from build123d import *

# Parameters (mm, degrees)
ESBO_O1_R                   = 16
RESSALTO_EXTRUS_O1_DEPTH    = 42
CASCA1_T                    = -5
ESBO_O3_R                   = 2
ESBO_O3_W                   = 60
ESBO_O3_H                   = 15
CORTE_EXTRUS_O1_DEPTH       = 5
ESBO_O4_R                   = 29
ESBO_O4_R_2                 = 24
RESSALTO_EXTRUS_O2_DEPTH    = 9
ESBO_O5_R                   = 9
CORTE_EXTRUS_O2_DEPTH       = 5
ESBO_O6_R                   = 14.5
ESBO_O6_R_2                 = 11.5
RESSALTO_EXTRUS_O3_DEPTH    = 6
NERVURA1_REACH              = 150.27
ESBO_O7_WALLS_W             = 304.540047886
ESBO_O7_WALLS_H             = 10
ESBO_O7_WALLS_W_2           = 10
ESBO_O7_WALLS_H_2           = 304.540047886
NERVURA2_REACH              = 150.866
ESBO_O8_WALLS_W             = 320.231422594
ESBO_O8_WALLS_H             = 10
ESBO_O8_WALLS_W_2           = 10
ESBO_O8_WALLS_H_2           = 400.231422594
ESBO_O8_WALLS_H_3           = 336.231422594
CORTE_EXTRUS_O3_DEPTH       = 5
ESBO_O10_R                  = 1.2
CORTE_EXTRUS_O4_DEPTH       = 5
RESSALTO_EXTRUS_O4_DEPTH    = 4
FILETE1_R                   = 1.5
PADR_O_LINEAR1_COUNT        = 3
PADR_O_LINEAR1_PITCH        = 65
FILETE1_OF_PADR_O_LINEAR1_R = 1.5


with BuildPart() as part:
    # Esboço1 → Ressalto-extrusão1 (new body)
    with BuildSketch(Plane.XY):
        with BuildLine():
            Line((-40, -100), (-40, 100))
            Line((-40, 100), (40, 100))
            Line((40, 100), (40, -100))
            ThreePointArc((40, -100), (0, -140), (-40, -100))
        make_face()
        with Locations(Location((0, -100, 0), (0, 0, 180))):
            Circle(ESBO_O1_R, mode=Mode.SUBTRACT)
    extrude(amount=RESSALTO_EXTRUS_O1_DEPTH)

    # Casca1
    casca1_openings = [part.faces().sort_by_distance(p)[0] for p in [
        (0, -12.059912395, 42),
        (16, -100, 21),
    ]]
    offset(amount=CASCA1_T, openings=casca1_openings, kind=Kind.INTERSECTION)

    # Esboço3 → Corte-extrusão1 (cut)
    with BuildSketch(Plane(origin=(0, 100, 0), x_dir=(1, 0, 0), z_dir=(0, 1, 0))):
        with Locations(Location((25, -33.5, 0), (0, 0, 270))):
            Circle(ESBO_O3_R)
        with Locations(Location((-25, -33.5, 0), (0, 0, 270))):
            Circle(ESBO_O3_R)
        with Locations(Location((-25, -8.5, 0), (0, 0, 270))):
            Circle(ESBO_O3_R)
        with Locations(Location((25, -8.5, 0), (0, 0, 270))):
            Circle(ESBO_O3_R)
        with Locations((0, -21)):
            Rectangle(ESBO_O3_W, ESBO_O3_H)
    extrude(amount=-CORTE_EXTRUS_O1_DEPTH, mode=Mode.SUBTRACT)

    # Esboço4 → Ressalto-extrusão2 (add)
    with BuildSketch(Plane.XY.offset(5)):
        with Locations((0, -100)):
            Circle(ESBO_O4_R)
        with Locations((0, -100)):
            Circle(ESBO_O4_R_2, mode=Mode.SUBTRACT)
    extrude(amount=RESSALTO_EXTRUS_O2_DEPTH)

    # Esboço5 → Corte-extrusão2 (cut)
    with BuildSketch(Plane.XY.offset(5)):
        with Locations((0, -20)):
            Circle(ESBO_O5_R)
    extrude(amount=-CORTE_EXTRUS_O2_DEPTH, mode=Mode.SUBTRACT)

    # Esboço6 → Ressalto-extrusão3 (add)
    with BuildSketch(Plane.XY.offset(5)):
        with Locations((0, -20)):
            Circle(ESBO_O6_R)
        with Locations((0, -20)):
            Circle(ESBO_O6_R_2, mode=Mode.SUBTRACT)
    extrude(amount=RESSALTO_EXTRUS_O3_DEPTH)

    # Esboço7 walls → Nervura1 (add, up to next)
    with BuildSketch(Plane.XY.offset(14), mode=Mode.PRIVATE) as nervura1_sk1:
        with Locations((32, -100)):
            Rectangle(ESBO_O7_WALLS_W, ESBO_O7_WALLS_H)
    nervura1_tool1 = extrude(nervura1_sk1.sketch, amount=-NERVURA1_REACH, mode=Mode.PRIVATE) - part.part
    # Esboço7 walls → Nervura1 (add, up to next)
    with BuildSketch(Plane.XY.offset(14), mode=Mode.PRIVATE) as nervura1_sk2:
        with Locations((-32, -100)):
            Rectangle(ESBO_O7_WALLS_W, ESBO_O7_WALLS_H)
    nervura1_tool2 = extrude(nervura1_sk2.sketch, amount=-NERVURA1_REACH, mode=Mode.PRIVATE) - part.part
    # Esboço7 walls → Nervura1 (add, up to next)
    with BuildSketch(Plane.XY.offset(14), mode=Mode.PRIVATE) as nervura1_sk3:
        with Locations((0, -132)):
            Rectangle(ESBO_O7_WALLS_W_2, ESBO_O7_WALLS_H_2)
    nervura1_tool3 = extrude(nervura1_sk3.sketch, amount=-NERVURA1_REACH, mode=Mode.PRIVATE) - part.part
    add(nervura1_tool1.solids().sort_by_distance((32, -100, 14))[0])
    add(nervura1_tool2.solids().sort_by_distance((-32, -100, 14))[0])
    add(nervura1_tool3.solids().sort_by_distance((0, -132, 14))[0])

    # Esboço8 walls → Nervura2 (add, up to next)
    with BuildSketch(Plane.XY.offset(11), mode=Mode.PRIVATE) as nervura2_sk1:
        with Locations((24.75, -20)):
            Rectangle(ESBO_O8_WALLS_W, ESBO_O8_WALLS_H)
    nervura2_tool1 = extrude(nervura2_sk1.sketch, amount=-NERVURA2_REACH, mode=Mode.PRIVATE) - part.part
    # Esboço8 walls → Nervura2 (add, up to next)
    with BuildSketch(Plane.XY.offset(11), mode=Mode.PRIVATE) as nervura2_sk2:
        with Locations((-24.75, -20)):
            Rectangle(ESBO_O8_WALLS_W, ESBO_O8_WALLS_H)
    nervura2_tool2 = extrude(nervura2_sk2.sketch, amount=-NERVURA2_REACH, mode=Mode.PRIVATE) - part.part
    # Esboço8 walls → Nervura2 (add, up to next)
    with BuildSketch(Plane.XY.offset(11), mode=Mode.PRIVATE) as nervura2_sk3:
        with Locations((0, 44.75)):
            Rectangle(ESBO_O8_WALLS_W_2, ESBO_O8_WALLS_H_2)
    nervura2_tool3 = extrude(nervura2_sk3.sketch, amount=-NERVURA2_REACH, mode=Mode.PRIVATE) - part.part
    # Esboço8 walls → Nervura2 (add, up to next)
    with BuildSketch(Plane.XY.offset(11), mode=Mode.PRIVATE) as nervura2_sk4:
        with Locations((0, -52.75)):
            Rectangle(ESBO_O8_WALLS_W_2, ESBO_O8_WALLS_H_3)
    nervura2_tool4 = extrude(nervura2_sk4.sketch, amount=-NERVURA2_REACH, mode=Mode.PRIVATE) - part.part
    add(nervura2_tool1.solids().sort_by_distance((24.75, -20, 11))[0])
    add(nervura2_tool2.solids().sort_by_distance((-24.75, -20, 11))[0])
    add(nervura2_tool3.solids().sort_by_distance((0, 44.75, 11))[0])
    add(nervura2_tool4.solids().sort_by_distance((0, -52.75, 11))[0])

    # Esboço9 → Corte-extrusão3 (cut)
    with BuildSketch(Plane.XY.offset(5)):
        with BuildLine():
            Line((-27.5, -52), (-12.5, -52))
            ThreePointArc((-12.5, -52), (-9.5, -55), (-12.5, -58))
            Line((-12.5, -58), (-27.5, -58))
            ThreePointArc((-27.5, -58), (-30.5, -55), (-27.5, -52))
        make_face()
    extrude(amount=-CORTE_EXTRUS_O3_DEPTH, mode=Mode.SUBTRACT)

    # Esboço10 → Corte-extrusão4 (cut)
    with BuildSketch(Plane.XY.offset(5)):
        with Locations((21.538461538, -66.293996461)):
            Circle(ESBO_O10_R)
        with Locations((28.694536951, -60.045749932)):
            Circle(ESBO_O10_R)
        Polygon((14.683545029, -56.348769838), (22.216255989, -49.771668228), (19.585415345, -46.758583844), (12.052704385, -53.335685454), align=None)
    extrude(amount=-CORTE_EXTRUS_O4_DEPTH, mode=Mode.SUBTRACT)

    # Esboço11 → Ressalto-extrusão4 (add)
    with BuildSketch(Plane(origin=(0, -65, 0), x_dir=(-1, 0, 0), z_dir=(0, -1, 0))):
        Polygon((-40, -21), (-31, -21), (-31, -36), (-33, -36), (-33, -26), (-40, -26), align=None)
    ressalto_extrus_o4 = extrude(amount=RESSALTO_EXTRUS_O4_DEPTH)

    # Filete1
    # the kernel refuses this fillet: 1.5 mm, written as the material it takes off along each edge
    with BuildSketch(Plane(origin=(31, -61.25, 21), x_dir=(1, 0, 0), z_dir=(0, -1, 0)), Plane(origin=(31, -61.25, 36), x_dir=(0, 0, -1), z_dir=(0, -1, 0))) as filete1_piece_1:
        with BuildLine():
            CenterArc((FILETE1_R, FILETE1_R), FILETE1_R, 180, 90)
            Line((0, FILETE1_R), (0, 0))
            Line((0, 0), (FILETE1_R, 0))
        make_face()
    extrude(amount=11.5, mode=Mode.SUBTRACT)
    with BuildSketch(Plane(origin=(33, -61.25, 36), x_dir=(0, 0, -1), z_dir=(0, -1, 0))) as filete1_piece_2:
        with BuildLine():
            CenterArc((FILETE1_R, -FILETE1_R), FILETE1_R, 90, 90)
            Line((0, -FILETE1_R), (0, 0))
            Line((0, 0), (FILETE1_R, 0))
        make_face()
    extrude(amount=11.5, mode=Mode.SUBTRACT)

    # Padrão linear1: Ressalto-extrusão4 ×3
    with Locations(*[(0, i * PADR_O_LINEAR1_PITCH, 0) for i in range(1, PADR_O_LINEAR1_COUNT)]):
        add(ressalto_extrus_o4)

    # Filete1 of Padrão linear1
    # the kernel refuses this fillet: 1.5 mm, written as the material it takes off along each edge
    with BuildSketch(Plane(origin=(31, 3.75, 21), x_dir=(1, 0, 0), z_dir=(0, -1, 0)), Plane(origin=(31, 3.75, 36), x_dir=(0, 0, -1), z_dir=(0, -1, 0)), Plane(origin=(31, 68.75, 21), x_dir=(1, 0, 0), z_dir=(0, -1, 0)), Plane(origin=(31, 68.75, 36), x_dir=(0, 0, -1), z_dir=(0, -1, 0))) as filete1_of_padr_o_linear1_piece_1:
        with BuildLine():
            CenterArc((FILETE1_OF_PADR_O_LINEAR1_R, FILETE1_OF_PADR_O_LINEAR1_R), FILETE1_OF_PADR_O_LINEAR1_R, 180, 90)
            Line((0, FILETE1_OF_PADR_O_LINEAR1_R), (0, 0))
            Line((0, 0), (FILETE1_OF_PADR_O_LINEAR1_R, 0))
        make_face()
    extrude(amount=11.5, mode=Mode.SUBTRACT)
    with BuildSketch(Plane(origin=(33, 3.75, 36), x_dir=(0, 0, -1), z_dir=(0, -1, 0)), Plane(origin=(33, 68.75, 36), x_dir=(0, 0, -1), z_dir=(0, -1, 0))) as filete1_of_padr_o_linear1_piece_2:
        with BuildLine():
            CenterArc((FILETE1_OF_PADR_O_LINEAR1_R, -FILETE1_OF_PADR_O_LINEAR1_R), FILETE1_OF_PADR_O_LINEAR1_R, 90, 90)
            Line((0, -FILETE1_OF_PADR_O_LINEAR1_R), (0, 0))
            Line((0, 0), (FILETE1_OF_PADR_O_LINEAR1_R, 0))
        make_face()
    extrude(amount=11.5, mode=Mode.SUBTRACT)


solid = part.part
Could you check a few things on this model? Use its own coordinates, in mm. A direction names the side the tool comes from. Give positions to 0.01 mm unless a question says otherwise; leave off trailing zeros. Write each loop counter-clockwise with the first axis right and the second up, starting at its lowest first coordinate (ties: lowest second). Pieces come first, ordered by that corner, then holes. Notation, with made-up numbers: (44, 84) -> (78, 84) arc R3 ccw to (78, 89) -> close; hole circle Ø7 at (-34.75, -24). An arc over 180 degrees is marked (long way). Answer as a JSON object with one key per item and string values.
Q1. Will these pins go through, and if not, where does the flat tip stop? pin 1 Ø1 at (x, y) = (-29, -78) entering from +Z; pin 2 Ø6.5 at (y, z) = (-130, 10.5) entering from +X; pin 3 Ø24 at (x, y) = (-21, -68) entering from +Z.
Taken from the geometry:
{"pin 1": "stops at z = 5", "pin 2": "stops at x = 29.74", "pin 3": "stops at z = 14"}
Q2. We'd pull the mould along Y, two halves only. Please class faces 4 (the cylindrical face through (0.77, -134.99, 23.24)), 5 (the flat face through (0, 98, 28.5)): released by +Y, released by -Y, zero draft, split by the parting line, or undercut.
Taken from the geometry:
{"face 4": "undercut", "face 5": "zero draft"}
Q3. Suppose I cut it at B-B on y = 23.5. Write out the boundary of the cut face in (x, z).
Taken from the geometry:
{"outline": "(-40, 0) -> (40, 0) -> (40, 42) -> (35, 42) -> (35, 5) -> (5, 5) -> (5, 11) -> (-5, 11) -> (-5, 5) -> (-35, 5) -> (-35, 42) -> (-40, 42) -> close"}
Q4. Suppose I cut it at C-C on z = 18.5. Write out the boundary of the cut face in (x, y), then the cut area to 3 significant figures.
Taken from the geometry:
{"outline": "(-40, -100) arc R40 ccw to (40, -100) -> (40, 100) -> (30, 100) -> (30, 95) -> (35, 95) -> (35, -100) arc R35 cw to (-35, -100) -> (-35, 95) -> (-30, 95) -> (-30, 100) -> (-40, 100) -> close", "area": "2,640 mm²"}
Q5. Please list where these lines run through material, in increasing order: L1, parallel to Y at x = 0, z = 1.5; L2, parallel to X at y = 63.5, z = 18.5; L3, parallel to X at y = 96.6, z = 8.5.
Taken from the geometry:
{"L1": "y = -140 to -116, -84 to -29, -11 to 100", "L2": "x = -40 to -35, 35 to 40", "L3": "x = -40 to -27, -23 to 23, 27 to 40"}
Q6. Suppose I cut it at A-A on y = -20. Write out the boundary of the cut face in (x, z).
Taken from the geometry:
{"outline": "(-40, 0) -> (-9, 0) -> (-9, 5) -> (-11.5, 5) -> (-11.5, 11) -> (-35, 11) -> (-35, 42) -> (-40, 42) -> close; (9, 0) -> (40, 0) -> (40, 42) -> (35, 42) -> (35, 11) -> (11.5, 11) -> (11.5, 5) -> (9, 5) -> close"}
Q7. Which directions (+Z, -Z, +X, -X, +Y, -Y) give clear straight access to the entire face, cutting with the end or side of a thin tool? Please do faces 1 (the flat face through (0, 98, 13.5)), 2 (the flat face through (-35, -4, 23)), 3 (the flat face through (-20, -52, 3)).
Taken from the geometry:
{"face 1": "+Y", "face 2": "+Z", "face 3": "+Z, -Z"}
